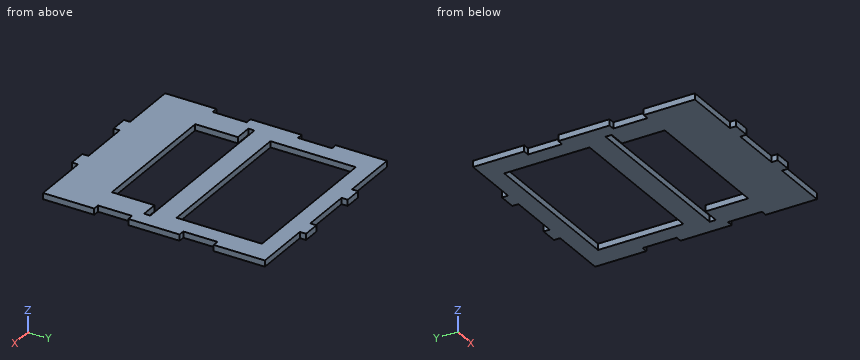
from build123d import *

# Parameters (mm, degrees)
SKETCH1_W           = 148.844
SKETCH1_H           = 174.244
BOSS_EXTRUDE1_DEPTH = 4.572
SKETCH2_W           = 42.672
SKETCH2_H           = 4.572
SKETCH2_W_2         = 38.1
CUT_EXTRUDE1_DEPTH  = 45.72
SKETCH3_W           = 4.572
SKETCH3_H           = 25.4
CUT_EXTRUDE2_DEPTH  = 45.72
SKETCH4_W           = 114.3
SKETCH4_H           = 63.5
SKETCH4_W_2         = 101.6
SKETCH4_H_2         = 31.75
CUT_EXTRUDE3_DEPTH  = 4.572
SKETCH5_W           = 127
SKETCH5_H           = 4.572
CUT_EXTRUDE4_DEPTH  = 4.572


with BuildPart() as part:
    # Sketch1 → Boss-Extrude1 (new body)
    with BuildSketch(Plane.XY):
        with Locations((74.422, 87.122)):
            Rectangle(SKETCH1_W, SKETCH1_H)
    extrude(amount=BOSS_EXTRUDE1_DEPTH)

    # Sketch2 → Cut-Extrude1 (cut)
    with BuildSketch(Plane.XY.offset(4.572)):
        with Locations((21.336, 2.286)):
            Rectangle(SKETCH2_W, SKETCH2_H)
        with Locations((74.422, 2.286)):
            Rectangle(SKETCH2_W_2, SKETCH2_H)
        with Locations((127.508, 2.286)):
            Rectangle(SKETCH2_W, SKETCH2_H)
        with Locations((21.336, 171.958)):
            Rectangle(SKETCH2_W, SKETCH2_H)
        with Locations((127.508, 171.958)):
            Rectangle(SKETCH2_W, SKETCH2_H)
        with Locations((74.422, 171.958)):
            Rectangle(SKETCH2_W_2, SKETCH2_H)
    extrude(amount=-CUT_EXTRUDE1_DEPTH, mode=Mode.SUBTRACT)

    # Sketch3 → Cut-Extrude2 (cut)
    with BuildSketch(Plane.XY.offset(4.572)):
        with Locations((146.558, 55.372)):
            Rectangle(SKETCH3_W, SKETCH3_H)
        with Locations((2.286, 55.372)):
            Rectangle(SKETCH3_W, SKETCH3_H)
        with Locations((146.558, 118.872)):
            Rectangle(SKETCH3_W, SKETCH3_H)
        with Locations((2.286, 118.872)):
            Rectangle(SKETCH3_W, SKETCH3_H)
    extrude(amount=-CUT_EXTRUDE2_DEPTH, mode=Mode.SUBTRACT)

    # Sketch4 → Cut-Extrude3 (cut)
    with BuildSketch(Plane(origin=(0, 0, 0), x_dir=(-1, 0, 0), z_dir=(0, 0, -1))):
        with Locations((-74.422, 125.222)):
            Rectangle(SKETCH4_W, SKETCH4_H)
        with Locations((-74.422, 57.277)):
            Rectangle(SKETCH4_W_2, SKETCH4_H_2)
    extrude(amount=-CUT_EXTRUDE3_DEPTH, mode=Mode.SUBTRACT)

    # Sketch5 → Cut-Extrude4 (cut)
    with BuildSketch(Plane(origin=(0, 0, 0), x_dir=(-1, 0, 0), z_dir=(0, 0, -1))):
        with Locations((-74.422, 75.438)):
            Rectangle(SKETCH5_W, SKETCH5_H)
    extrude(amount=-CUT_EXTRUDE4_DEPTH, mode=Mode.SUBTRACT)


solid = part.part
The listing builds one solid part. Answer for the finished solid, in the listing's coordinates (mm). Give positions to 0.01 mm unless a question says otherwise; leave off trailing zeros. Write each loop counter-clockwise with the first axis right and the second up, starting at its lowest first coordinate (ties: lowest second). Pieces come first, ordered by that corner, then holes. Notation, with made-up numbers: (-5, 84) - (40, 84) arc R22 cw to (40, 117) - close; hole circle Ø3 at (37.5, 47.25). An arc over 180 degrees is marked (long way). Use a Markdown table: item, result.
1. Find the intervals of material crossed by probe 1 along Y at (x, z) = (50, 0.85); probe 2 along Y at (x, z) = (83, 0.3); probe 3 along X at (y, z) = (128, 1.7), in increasing order. Write a range as from..to.
Values follow:
| item | result |
|---|---|
| probe 1 | y = 0..41.4, 77.72..93.47, 156.97..174.24 |
| probe 2 | y = 4.57..41.4, 77.72..93.47, 156.97..169.67 |
| probe 3 | x = 4.57..17.27, 131.57..144.27 |
2. Each of these flat-tipped pins is pushed along its axis until it touches: P1, Ø2.5, axis at y = 52.5, z = 1.5, coming from the +X side; P2, Ø2, axis at y = 53, z = 3.5, coming from the -X side; P3, Ø1.4, axis at y = 2, z = 3.5, coming from the +X side; P4, Ø3, axis at x = 22, y = 46, coming from the -Z side. Where does it stop, or does it pass through?
Values follow:
| item | result |
|---|---|
| P1 | stops at x = 144.27 |
| P2 | stops at x = 4.57 |
| P3 | stops at x = 106.17 |
| P4 | stops at z = 0 |
3. Section C-C on z = 1.2 is taken. Count the separate pieces of the cut face and the enclosed holes in it, plus the area to 3 significant figures.
Values follow:
| item | result |
|---|---|
| separate pieces | 1 |
| enclosed holes | 2 |
| area | 13,300 mm² |
4. Section B-B on y = 121 is taken. Write down the section's boundary in (x, z).
Values follow:
| item | result |
|---|---|
| outline | (4.57, 0) - (17.27, 0) - (17.27, 4.57) - (4.57, 4.57) - close; (131.57, 0) - (144.27, 0) - (144.27, 4.57) - (131.57, 4.57) - close |
5. Section A-A on x = 60.5 is taken. Write down the section's boundary in (y, z).
Values follow:
| item | result |
|---|---|
| outline | (4.57, 0) - (41.4, 0) - (41.4, 4.57) - (4.57, 4.57) - close; (77.72, 0) - (93.47, 0) - (93.47, 4.57) - (77.72, 4.57) - close; (156.97, 0) - (169.67, 0) - (169.67, 4.57) - (156.97, 4.57) - close |
6. Section D-D on y = 140 is taken. Write down the section's boundary in (x, z).
Values follow:
| item | result |
|---|---|
| outline | (0, 0) - (17.27, 0) - (17.27, 4.57) - (0, 4.57) - close; (131.57, 0) - (148.84, 0) - (148.84, 4.57) - (131.57, 4.57) - close |
